The listing builds one solid part. Answer for the finished solid, in the listing's coordinates (mm). A direction names the side the tool comes from. Coordinates: 2 decimals unless noted, no trailing zeros. Order: outer loops, then holes, each group sorted by start corner. A loop starts at its lowest first (then second) coordinate and runs counter-clockwise, first axis right, second up. Notation, with made-up numbers: (43.25, 32.25) -> (85.25, 32.25) arc R26 ccw to (85.25, 64.25) -> close; hole circle Ø10 at (-38, 67). An arc over 180 degrees is marked (long way). Answer in a Markdown table with one row per item.
```python
from build123d import *

# Parameters (mm, degrees)
SKETCH1_W           = 70
SKETCH1_H           = 70
BOSS_EXTRUDE2_DEPTH = 7
CUT_EXTRUDE1_DEPTH  = 5
SKETCH9_W           = 70
SKETCH9_H           = 70
BOSS_EXTRUDE3_DEPTH = 5
CUT_EXTRUDE11_DEPTH = 100.242128151
SKETCH21_R          = 3
CUT_EXTRUDE12_DEPTH = 2
CHAMFER3_SIZE       = 1
CUT_EXTRUDE13_START = -2
SKETCH22_W          = 70
SKETCH22_H          = 70
CUT_EXTRUDE13_DEPTH = 2
SKETCH27_R          = 3
CUT_EXTRUDE27_DEPTH = 2
SKETCH28_R          = 3
CUT_EXTRUDE28_DEPTH = 2


with BuildPart() as part:
    # Sketch1 → Boss-Extrude2 (new body)
    with BuildSketch(Plane(origin=(0, 0, 0), x_dir=(1, 0, 0), z_dir=(0, 1, 0))):
        with Locations((35, 35)):
            Rectangle(SKETCH1_W, SKETCH1_H)
    extrude(amount=BOSS_EXTRUDE2_DEPTH)

    # Sketch3 → Cut-Extrude1 (cut)
    with BuildSketch(Plane(origin=(0, 7, 0), x_dir=(1, 0, 0), z_dir=(0, 1, 0))):
        with BuildLine():
            Line((2.5, 57.5), (2.5, 12.5))
            ThreePointArc((2.5, 12.5), (5.428932188, 5.428932188), (12.5, 2.5))
            Line((12.5, 2.5), (57.5, 2.5))
            ThreePointArc((57.5, 2.5), (64.571067812, 5.428932188), (67.5, 12.5))
            Line((67.5, 12.5), (67.5, 57.5))
            ThreePointArc((67.5, 57.5), (64.571067812, 64.571067812), (57.5, 67.5))
            Line((57.5, 67.5), (12.5, 67.5))
            ThreePointArc((12.5, 67.5), (5.428932188, 64.571067812), (2.5, 57.5))
        make_face()
    extrude(amount=-CUT_EXTRUDE1_DEPTH, mode=Mode.SUBTRACT)

    # Sketch9 → Boss-Extrude3 (add)
    with BuildSketch(Plane.XZ):
        with Locations((35, -35)):
            Rectangle(SKETCH9_W, SKETCH9_H)
    extrude(amount=BOSS_EXTRUDE3_DEPTH)

    # Sketch20 → Cut-Extrude11 (cut, through all)
    with BuildSketch(Plane(origin=(0, 2, 0), x_dir=(1, 0, 0), z_dir=(0, 1, 0))):
        with BuildLine():
            Line((13.745191882, 7.5), (56.254808118, 7.5))
            ThreePointArc((56.254808118, 7.5), (57.5, 12.5), (62.5, 13.745191882))
            Line((62.5, 13.745191882), (62.5, 56.254808118))
            ThreePointArc((62.5, 56.254808118), (57.5, 57.5), (56.254808118, 62.5))
            Line((56.254808118, 62.5), (13.745191882, 62.5))
            ThreePointArc((13.745191882, 62.5), (12.5, 57.5), (7.5, 56.254808118))
            Line((7.5, 56.254808118), (7.5, 13.745191882))
            ThreePointArc((7.5, 13.745191882), (12.5, 12.5), (13.745191882, 7.5))
        make_face()
    extrude(amount=-CUT_EXTRUDE11_DEPTH, mode=Mode.SUBTRACT)

    # Sketch21 → Cut-Extrude12 (cut)
    with BuildSketch(Plane(origin=(0, 2, 0), x_dir=(1, 0, 0), z_dir=(0, 1, 0))):
        with Locations(Location((8.964466094, 61.035533906, 0), (0, 0, 270))):
            Circle(SKETCH21_R)
        with Locations(Location((61.035533906, 61.035533906, 0), (0, 0, 270))):
            Circle(SKETCH21_R)
        with Locations(Location((61.035533906, 8.964466094, 0), (0, 0, 270))):
            Circle(SKETCH21_R)
        with Locations(Location((8.964466094, 8.964466094, 0), (0, 0, 270))):
            Circle(SKETCH21_R)
    extrude(amount=-CUT_EXTRUDE12_DEPTH, mode=Mode.SUBTRACT)

    # Chamfer3
    chamfer3_edges = [part.edges().sort_by_distance(p)[0] for p in [
        (5.428932188, 7, -5.428932188),
        (35, 7, -2.5),
        (64.571067812, 7, -5.428932188),
        (67.5, 7, -35),
        (64.571067812, 7, -64.571067812),
        (35, 7, -67.5),
        (5.428932188, 7, -64.571067812),
        (2.5, 7, -35),
        (12.5, 2, -12.5),
        (12.5, 2, -57.5),
        (57.5, 2, -57.5),
        (57.5, 2, -12.5),
        (35, 2, -7.5),
        (62.5, 2, -35),
        (35, 2, -62.5),
        (7.5, 2, -35),
    ]]
    chamfer(chamfer3_edges, length=CHAMFER3_SIZE)

    # Sketch22 → Cut-Extrude13 (cut)
    with BuildSketch(Plane.XZ.offset(5).offset(CUT_EXTRUDE13_START)):
        with Locations((35, -35)):
            Rectangle(SKETCH22_W, SKETCH22_H)
        with BuildLine():
            Line((7.5, -13.745191882), (7.5, -56.254808118))
            ThreePointArc((7.5, -56.254808118), (12.5, -57.5), (13.745191882, -62.5))
            Line((13.745191882, -62.5), (56.254808118, -62.5))
            ThreePointArc((56.254808118, -62.5), (57.5, -57.5), (62.5, -56.254808118))
            Line((62.5, -56.254808118), (62.5, -13.745191882))
            ThreePointArc((62.5, -13.745191882), (57.5, -12.5), (56.254808118, -7.5))
            Line((56.254808118, -7.5), (13.745191882, -7.5))
            ThreePointArc((13.745191882, -7.5), (12.5, -12.5), (7.5, -13.745191882))
        make_face(mode=Mode.SUBTRACT)
    extrude(amount=CUT_EXTRUDE13_DEPTH, mode=Mode.SUBTRACT)

    # Sketch27 → Cut-Extrude27 (cut)
    with BuildSketch(Plane.ZY):
        with Locations((-62.5, 2)):
            Circle(SKETCH27_R)
        with Locations((-7.5, 2)):
            Circle(SKETCH27_R)
    cut_extrude27 = extrude(amount=-CUT_EXTRUDE27_DEPTH, mode=Mode.SUBTRACT)

    # Mirror4: Cut-Extrude27 across plane
    add(cut_extrude27.mirror(Plane.ZY.offset(-35)), mode=Mode.SUBTRACT)

    # Sketch28 → Cut-Extrude28 (cut)
    with BuildSketch(Plane.XY):
        with Locations((7.5, 2)):
            Circle(SKETCH28_R)
        with Locations((62.5, 2)):
            Circle(SKETCH28_R)
    cut_extrude28 = extrude(amount=-CUT_EXTRUDE28_DEPTH, mode=Mode.SUBTRACT)

    # Mirror5: Cut-Extrude28 across plane
    add(cut_extrude28.mirror(Plane.XY.offset(-35)), mode=Mode.SUBTRACT)


solid = part.part
```
(1) A cutting plane is placed at A-A, the plane z = -30.5. Determine the outline of the cut face in (x, y).
Check values:
| item | result |
|---|---|
| outline | (0, -3) -> (7.5, -3) -> (7.5, 1) -> (6.5, 2) -> (2.5, 2) -> (2.5, 6) -> (1.5, 7) -> (0, 7) -> close; (62.5, -3) -> (70, -3) -> (70, 7) -> (68.5, 7) -> (67.5, 6) -> (67.5, 2) -> (63.5, 2) -> (62.5, 1) -> close |
(2) Find the intervals of material crossed by line 1 along X through (y, z) = (0.25, -9); line 2 along Z through (x, y) = (55, 4.75); line 3 along X through (y, z) = (-1.5, -61), in increasing order. Write a range as from..to.
Check values:
| item | result |
|---|---|
| line 1 | 2..5.96, 11.96..13.96, 56.04..58.04, 64.04..68 |
| line 2 | -70..-67.5, -2.5..0 |
| line 3 | 0..13.96, 56.04..70 |
(3) Which of the six approach directions +Z, -Z, +X, -X, +Y, -Y give full straight-line access (tool end or side, diameter ignored) to faces 1 (the flat face through (62.5, -1, -35)), 2 (the flat face through (2, 2, -63)), 3 (the flat face through (9, 0, -61))?
Check values:
| item | result |
|---|---|
| face 1 | +Y, -Y |
| face 2 | -X |
| face 3 | +Y |
(4) Flat-ended cylindrical pins translate along their axes: pin 1 (6 mm diameter, centred on x = 15, z = -11, fed in from +Y); pin 2 (3.5 mm diameter, centred on y = 2, z = -62.5, fed in from -X); pin 3 (1.8 mm diameter, centred on y = 1, z = -7, fed in from +X). Find the tip coordinate at first contact, or state that the pin passes through.
Check values:
| item | result |
|---|---|
| pin 1 | y = 2 |
| pin 2 | x = 2 |
| pin 3 | x = 68 |
(5) A cutting plane is placed at B-B, the plane x = 25.5. Determine the outline of the cut face in (y, z).
Check values:
| item | result |
|---|---|
| outline | (-3, -70) -> (7, -70) -> (7, -68.5) -> (6, -67.5) -> (2, -67.5) -> (2, -63.5) -> (1, -62.5) -> (-3, -62.5) -> close; (-3, -7.5) -> (1, -7.5) -> (2, -6.5) -> (2, -2.5) -> (6, -2.5) -> (7, -1.5) -> (7, 0) -> (-3, 0) -> close |
(6) For a pull along Z with two mould halves and no side action, classify faces 4 (the cylindrical face through (10.36, 2.9, -0.99)), 5 (the flat face through (7.5, -1, -35)) as released by +Z, released by -Z, zero draft, split by the parting line, or undercut.
Check values:
| item | result |
|---|---|
| face 4 | zero draft |
| face 5 | undercut |
